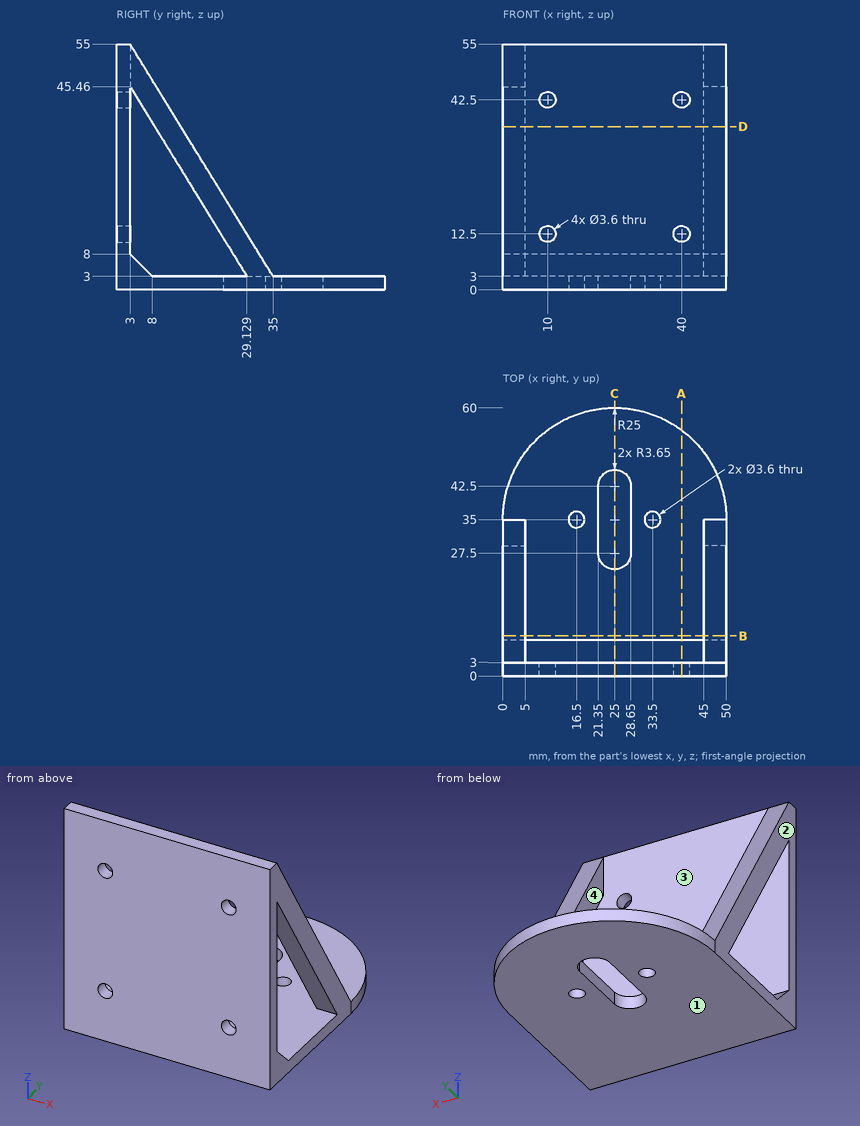
Job drawing, mm, ordinate dimensions from the low corner. One solid piece. Give positions to 0.01 mm unless a question says otherwise; leave off trailing zeros. Loops run counter-clockwise (first coordinate to the right, second up) from the corner with the lowest first, then second, coordinate; pieces in that order, holes last.
Item 1: Slice it at C-C, the plane x = 25. List the corners of the cut face in (y, z), and give its area (3 significant figures).
Answers follow:
outline: (0, 0) - (23.85, 0) - (23.85, 3) - (8, 3) - (3, 8) - (3, 55) - (0, 55) - close; (46.15, 0) - (60, 0) - (60, 3) - (46.15, 3) - close
area: 282 mm2
Item 2: Pull direction X, two halves, no side cores. Call the marked faces 1, 2, 3 and 4: released by +X, released by -X, zero draft, split by the parting line, or undercut.
Answers follow:
face 1: zero draft
face 2: released by -X
face 3: undercut
face 4: undercut
Item 3: Drill centre lines: line 1 (Z direction, x = 40, y = 1.15); line 2 (X direction, y = 5.5, z = 44.5); line 3 (Y direction, x = 6.5, z = 36). Where is each one in solid material? Low to high.
Answers follow:
line 1: z = 0 to 10.7, 14.3 to 40.7, 44.3 to 55
line 2: x = 0 to 5, 45 to 50
line 3: y = 0 to 3
Item 4: Slice it at B-B, the plane y = 9. List the corners of the cut face in (x, z), and give its area (3 significant figures).
Answers follow:
outline: (0, 0) - (50, 0) - (50, 3) - (0, 3) - close; (0, 35.71) - (5, 35.71) - (5, 45.25) - (0, 45.25) - close; (45, 35.71) - (50, 35.71) - (50, 45.25) - (45, 45.25) - close
area: 245 mm2
Item 5: Slice it at A-A, the plane x = 40. List the corners of the cut face in (y, z).
Answers follow:
outline: (0, 0) - (55, 0) - (55, 3) - (8, 3) - (3, 8) - (3, 10.7) - (0, 10.7) - close; (0, 14.3) - (3, 14.3) - (3, 40.7) - (0, 40.7) - close; (0, 44.3) - (3, 44.3) - (3, 55) - (0, 55) - close
Item 6: Slice it at D-D, the plane z = 36.5. List the corners of the cut face in (x, y) (1 decimal).
Answers follow:
outline: (0, 0) - (50, 0) - (50, 3) - (0, 3) - close; (0, 8.5) - (5, 8.5) - (5, 14.4) - (0, 14.4) - close; (45, 8.5) - (50, 8.5) - (50, 14.4) - (45, 14.4) - close
Item 7: Flat gauge pins, fed straight in: pin 1 (4.5 mm diameter, centred on x = 16.5, y = 35, fed in from -Z); pin 2 (8 mm diameter, centred on x = 31.5, y = 47, fed in from +Z); pin 3 (9.5 mm diameter, centred on y = 26.5, z = 33.5, fed in from -X); pin 4 (0.9 mm diameter, centred on y = 37.5, z = 1.5, fed in from -X). Where does each tip first touch, or does it go through?
Answers follow:
pin 1: stops at z = 0
pin 2: stops at z = 3
pin 3: passes through
pin 4: stops at x = 0.08
